```python
from build123d import *

# Parameters (mm, degrees)
EXTRUDE1_DEPTH  = 120
LPATTERN1_COUNT = 2
LPATTERN1_PITCH = 60


with BuildPart() as part:
    # Sketch1 → Extrude1 (new body)
    with BuildSketch(Plane(origin=(-20, 0, 0), x_dir=(1, 0, 0), z_dir=(0, 0, 1))):
        with BuildLine():
            Line((12.5, 0.69999271), (13.199992786, 0))
            Line((13.199992786, 0), (26.800007214, 0))
            Line((26.800007214, 0), (27.5, 0.69999271))
            Line((27.5, 0.69999271), (27.5, 4.2000246))
            Line((27.5, 4.2000246), (24.8000183, 6.9000063))
            Line((24.8000183, 6.9000063), (24.8000183, 8.8400054))
            Line((24.8000183, 8.8400054), (25.755946813, 9.794179118))
            ThreePointArc((25.755946813, 9.794179118), (26.198484624, 10.690600567), (27.09432569, 11.13431209))
            Line((27.09432569, 11.13431209), (27.5, 11.5399866))
            Line((27.5, 11.5399866), (27.5, 12.8500204))
            Line((27.5, 12.8500204), (27.09432569, 13.268442751))
            ThreePointArc((27.09432569, 13.268442751), (26.202460867, 13.706434947), (25.755946813, 14.594063938))
            Line((25.755946813, 14.594063938), (25.3500197, 15))
            Line((25.3500197, 15), (14.6499803, 15))
            Line((14.6499803, 15), (14.244053187, 14.594063938))
            ThreePointArc((14.244053187, 14.594063938), (13.797539133, 13.706434947), (12.90567431, 13.268442751))
            Line((12.90567431, 13.268442751), (12.5, 12.8500204))
            Line((12.5, 12.8500204), (12.5, 11.5399866))
            Line((12.5, 11.5399866), (12.90567431, 11.13431209))
            ThreePointArc((12.90567431, 11.13431209), (13.801515376, 10.690600567), (14.244053187, 9.794179118))
            Line((14.244053187, 9.794179118), (15.1999817, 8.8400054))
            Line((15.1999817, 8.8400054), (15.1999817, 6.9000063))
            Line((15.1999817, 6.9000063), (12.5, 4.2000246))
            Line((12.5, 4.2000246), (12.5, 0.69999271))
        make_face()
    extrude(amount=-EXTRUDE1_DEPTH)

    # Sketch2 → Cut-Revolve1 (revolve, cut)
    with BuildSketch(Plane(origin=(0, 0, 0), x_dir=(0, 0, -1), z_dir=(1, 0, 0))):
        Polygon((20, 15), (23.75, 15), (23.75, 9.7), (22.25, 9.7), (22.25, 0), (20, 0), align=None)
    cut_revolve1 = revolve(axis=Axis((0, 0, -20), (0, 1, 0)), mode=Mode.SUBTRACT)

    # LPattern1: Cut-Revolve1 ×2
    with Locations(*[(0, 0, -i * LPATTERN1_PITCH) for i in range(1, LPATTERN1_COUNT)]):
        add(cut_revolve1, mode=Mode.SUBTRACT)


solid = part.part
```
Verification items for the finished model (mm, model axes). A direction names the side the tool comes from. Coordinates: 2 decimals unless noted, no trailing zeros. Loops run counter-clockwise (first coordinate to the right, second up) from the corner with the lowest first, then second, coordinate; pieces in that order, holes last. Notation, with made-up numbers: (28.25, 21) -> (40.25, 21) arc R27 cw to (40.25, 43) -> close; hole circle Ø9 at (45.5, 64). An arc over 180 degrees is marked (long way). Put each result on its own line as item: value.
1. Thickness scan on line 1 (Z direction, x = 0, y = 2.5); line 2 (X direction, y = 12, z = -80); line 3 (Z direction, x = 0, y = 12). Record the ranges inside material, lowest first.
Result set:
line 1: z = -120 to -82.25, -77.75 to -22.25, -17.75 to 0
line 2: x = -7.5 to -3.75, 3.75 to 7.5
line 3: z = -120 to -83.75, -76.25 to -23.75, -16.25 to 0
2. Section check C-C, the plane y = 2.5. Record the boundary of the cut face in (x, z).
Result set:
outline: (-7.5, -120) -> (7.5, -120) -> (7.5, 0) -> (-7.5, 0) -> close; hole circle Ø4.5 at (0, -80); hole circle Ø4.5 at (0, -20)
3. Section check D-D, the plane z = -56. Record the boundary of the cut face in (x, y).
Result set:
outline: (-7.5, 0.7) -> (-6.8, 0) -> (6.8, 0) -> (7.5, 0.7) -> (7.5, 4.2) -> (4.8, 6.9) -> (4.8, 8.84) -> (5.76, 9.79) arc R1.56 cw to (7.09, 11.13) -> (7.5, 11.54) -> (7.5, 12.85) -> (7.09, 13.27) arc R1.56 cw to (5.76, 14.59) -> (5.35, 15) -> (-5.35, 15) -> (-5.76, 14.59) arc R1.56 cw to (-7.09, 13.27) -> (-7.5, 12.85) -> (-7.5, 11.54) -> (-7.09, 11.13) arc R1.56 cw to (-5.76, 9.79) -> (-4.8, 8.84) -> (-4.8, 6.9) -> (-7.5, 4.2) -> close
4. Section check A-A, the plane x = 0. Record the boundary of the cut face in (y, z).
Result set:
outline: (0, -120) -> (15, -120) -> (15, -83.75) -> (9.7, -83.75) -> (9.7, -82.25) -> (0, -82.25) -> close; (0, -77.75) -> (9.7, -77.75) -> (9.7, -76.25) -> (15, -76.25) -> (15, -23.75) -> (9.7, -23.75) -> (9.7, -22.25) -> (0, -22.25) -> close; (0, -17.75) -> (9.7, -17.75) -> (9.7, -16.25) -> (15, -16.25) -> (15, 0) -> (0, 0) -> close
5. Tool access check on faces 1 (the face through (6.2, 5.5, -59.2)), 2 (the face through (-0.165, 12.313, -16.254)), 3 (the face through (-6.1, 5.6, -59.2)). Record the directions out of +Z, -Z, +X, -X, +Y, -Y that give a thin tool (end or side, any length) a straight path to the whole face; none if there is none.
Result set:
face 1: +Z, -Z, +X
face 2: +Y
face 3: +Z, -Z, -X
6. Mould release check, pull along X, two halves, no side actions. Record for faces 4 (the face through (0, 8, -120)), 5 (the face through (-4.8, 8, -59)), 6 (the face through (4.8, 8, -59)), 7 (the face through (2, 9.7, -82)): pulls with the +X half, pulls with the -X half, needs draft (parallel to the pull), parting line crosses it, or undercut.
Result set:
face 4: needs draft
face 5: pulls with the -X half
face 6: pulls with the +X half
face 7: undercut
7. Gauge pin test, flat ends, axial feed: P1, Ø6, axis at x = 0, z = -80, coming from the +Y side; P2, Ø3.5, axis at x = 0, z = -20, coming from the +Y side; P3, Ø4, axis at y = 6.5, z = -60.5, coming from the +X side; P4, Ø1, axis at y = 7.5, z = -43, coming from the +X side. Record the tip position at first contact, or that the pin passes through.
Result set:
P1: stops at y = 9.7
P2: passes through
P3: stops at x = 7.2
P4: stops at x = 4.8
